from build123d import *

# Parameters (mm, degrees)
F1_DEPTH = 150
F2_DEPTH = 15
F2_TAPER = -45


with BuildPart() as f1:
    # F0 (on Front) → F1 (new body)
    with BuildSketch(Plane.XZ):
        Polygon((5.5549415993, 5.1121377619), (0.7767878706, -1.1757001048), (-7.1085173404, 2.4076352129), (0.7767878706, -6.34407287), align=None)
    extrude(amount=F1_DEPTH)

    # F1_face (on face) → F2 (join)
    with BuildSketch(Plane(origin=(-0.2589292902, 0, -1.3638932288), x_dir=(1, 0, 0), z_dir=(0, 1, 0))):
        Polygon((1.0357171608, 4.9801796412), (-6.8495880502, -3.7715284417), (1.0357171608, -0.188193124), (5.8138708894, -6.4760309907), align=None)
    extrude(amount=F2_DEPTH, taper=F2_TAPER)


solid = f1.part
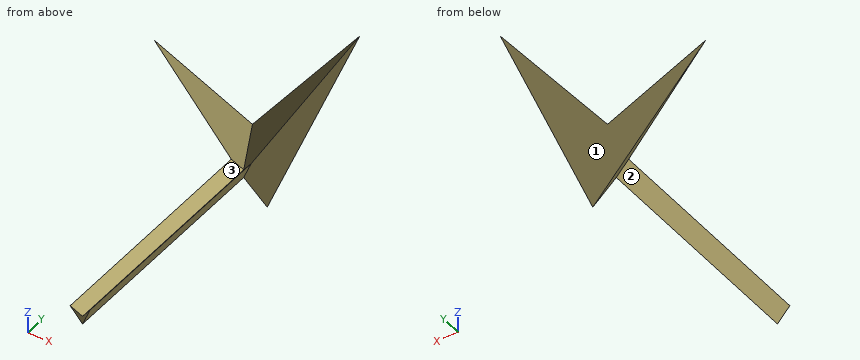
CAD build for the part. Positions are in the model's coordinates, mm. Face numbers are marked on the shaded views. Coordinates: 2 decimals unless noted, no trailing zeros. Order: outer loops, then holes, each group sorted by start corner. A loop starts at its lowest first (then second) coordinate and runs counter-clockwise, first axis right, second up.
Item 1: Drill centre lines: L1, parallel to X at y = -117, z = 0; L2, parallel to Y at x = 16, z = 0.5. Where is each one in solid material? Low to high.
Check sheet entries:
L1: x = -4.94 to -1.81, 1.67 to 3.42
L2: y = 11.42 to 15
Item 2: Band-saw the part on A-A on y = -111.5. List the corners of the cut face in (x, z), plus the area to 3 significant figures.
Check sheet entries:
outline: (-7.11, 2.41) - (0.78, -6.34) - (5.55, 5.11) - (0.78, -1.18) - close
area: 32.7 mm2
Item 3: Two-plate mould, pull along X, no slides. Class the marked faces 1, 2 and 3: +X half, -X half, draft (parallel to the pull), parting line (faces both ways), or undercut.
Check sheet entries:
face 1: draft
face 2: -X half
face 3: undercut
